Here's how the part is built. I have some questions about the finished solid (model axes, mm). A direction names the side the tool comes from. Coordinates: 2 decimals unless noted, no trailing zeros. Write each loop counter-clockwise with the first axis right and the second up, starting at its lowest first coordinate (ties: lowest second). Pieces come first, ordered by that corner, then holes. Notation, with made-up numbers: (70, 31) - (107, 31) arc R16 ccw to (107, 46) - close; hole circle Ø8 at (51.5, -34). An arc over 180 degrees is marked (long way). Answer in a Markdown table with one row per item. Add a question column.
Item 1: I'm going to push flat-ended pins straight in: pin 1 (6 mm diameter, centred on x = -9, y = -2, fed in from -Z); pin 2 (0.5 mm diameter, centred on y = 0, z = -3.5, fed in from -X); pin 3 (1 mm diameter, centred on x = 8.5, z = 0, fed in from -Y). Where does each tip first touch, or does it pass through?
Item 2: Imagine slicing it at B-B (y = -4.5). Please give me the cut outline in (x, z).
Item 3: We'd pull the mould along X, two halves only. Please class faces 3 (the face through (-6.096, 0, -3.6)), 4 (the face through (9.761, 1.699, 3.267)), 5 (the face through (2.842, 1.699, 3.267)), 6 (the face through (5.027, 3.436, 1.424)): +X half, -X half, draft (parallel to the pull), parting line (faces both ways), or undercut.
Item 4: Imagine slicing it at C-C (x = 5). Please give me the cut outline in (y, z), plus the area to 3 significant figures.
Item 5: If I drill on probe 1 along Y at (x, z) = (-0.95, 0); probe 2 along X at (y, z) = (1.5, -1.75); probe 3 along X at (y, z) = (-2, 1.5), over which ranges is the centre line in solid material (lowest first)? Write a range as from..to.
Item 6: Imagine slicing it at A-A (x = 7.5). Please give me the cut outline in (y, z).
Item 7: Which directions (+Z, -Z, +X, -X, +Y, -Y) give clear straight access to the entire face, cutting with the end or side of a thin tool? Please do faces 1 (the face through (-8.6, -0.508, 3.5)), 2 (the face through (0, -2, 4)).
Autodesk Inventor part; units mm, degrees
ref_plane "YZ Plane" through (0, 0, 0) normal (1, 0, 0) x (0, 1, 0)
ref_plane "XZ Plane" through (0, 0, 0) normal (0, 1, 0) x (-1, 0, 0)
ref_plane "XY Plane" through (0, 0, 0) normal (0, 0, 1) x (1, 0, 0)
sketch "Sketch1" plane through (0, 0, 0) normal (0, 0, 1) x (1, 0, 0)
  line L0 (0, 0) -> (1.778, 0)
  line L1 (1.778, 0) -> (1.778, 5.08)
  line L2 (1.778, 5.08) -> (0, 5.08)
  line L3 (0, 5.08) -> (0, 0)
  line L4 (1.778, 0) -> (11.049, 0)
  line L5 (11.049, 0) -> (11.049, 3.683)
  line L6 (11.049, 3.683) -> (1.778, 3.683)
  line L7 (1.778, 3.683) -> (1.778, 0)
  line L8 (8.509, 3.683) -> (6.985, 3.81)
  line L9 (6.985, 3.81) -> (6.985, 3.683)
  line L10 (6.985, 3.683) -> (5.461, 3.81)
  line L11 (5.461, 3.81) -> (5.461, 3.683)
  line L12 (5.461, 3.683) -> (3.937, 3.81)
  line L13 (3.937, 3.81) -> (3.937, 3.683)
  line L14 (0, 0) -> (0, 3.1252)
  line L15 (0, 4.191) -> (0.889, 4.191) construction
  line L16 (0, 4.191) -> (0, 0)
  arc A0 (0, 4.191) -> (-9.906, 3.937) centre (0, -189.103) ccw
  line L17 (-9.906, 3.937) -> (-9.906, 4.191)
  line L18 (-9.906, 4.191) -> (-11.176, 4.191)
  line L19 (-11.176, 4.191) -> (-11.176, 0)
  line L20 (-11.176, 0) -> (0, 0)
  dimension "d0" = 1.778
  dimension "d1" = 10.16
  dimension "d2" = 9.271
  dimension "d3" = 7.366
  dimension "d4" = 7.62
  dimension "d5" = 2.54
  dimension "d6" = 1.524
  dimension "d7" = 8.382
  dimension "d8" = 8.382
  dimension "d9" = 11.176
  dimension "d10" = 7.874
  dimension "d11" = 1.27
revolve "Revolution1" add sketch "Sketch1" angle 360 about axis through (-11.176, 0, 0) along (1, 0, 0)
sketch "Sketch2" plane through (0, 0, 0) normal (0, 0, 1) x (1, 0, 0)
  line L0 (-11.176, 0.508) -> (-6.096, 0.508)
  line L1 (-6.096, 0.508) -> (-6.096, -0.508)
  line L2 (-6.096, -0.508) -> (-11.176, -0.508)
  line L3 (-11.176, -0.508) -> (-11.176, 0.508)
  line L4 (-11.176, -4.191) -> (-11.176, 4.191) construction
  point P0 (0, 0)
  point P1 (-11.176, 0)
  dimension "d13" = 1.016
  dimension "d14" = 5.08
extrude "Extrusion1" cut sketch "Sketch2" along normal through all both and the other way through all
hole "Hole1" at (-11.176, 0, 0) direction (1, 0, 0) diameter 4.7625 depth 11.1125 counterbore diameter 6.35 counterbore depth 6.35
hole "Hole2" at (11.049, 0, 0) direction (-1, 0, 0) diameter 4.7625 depth 9.525 counterbore diameter 6.35 counterbore depth 1.27
equation "\"d8\" = d7"
properties part number "T9 Axle"
Here are the results:
| question | item | result |
|---|---|---|
| 1 | pin 1 | stops at z = -4.16 |
| 1 | pin 2 | stops at x = -6.1 |
| 1 | pin 3 | stops at y = -3.73 |
| 2 | outline | (0, -2.36) - (1.78, -2.36) - (1.78, 2.36) - (0, 2.36) - close |
| 3 | face 3 | -X half |
| 3 | face 4 | draft |
| 3 | face 5 | undercut |
| 3 | face 6 | undercut |
| 4 | outline | circle Ø7.44 at (0, 0); hole circle Ø4.76 at (0, 0) |
| 4 | area | 25.7 mm2 |
| 5 | probe 1 | y = -4.19..-2.38, 2.38..4.19 |
| 5 | probe 2 | x = -0.06..1.52 |
| 5 | probe 3 | x = -4.83..9.78 |
| 6 | outline | circle Ø7.53 at (0, 0); hole circle Ø4.76 at (0, 0) |
| 7 | face 1 | +Z, -Z, -X |
| 7 | face 2 | -X |
